Answer from the drawing. Dimensions are ordinates in mm from the lowest x, y and z of the part. A direction names the side the tool comes from. Round coordinates to 2 decimals unless told otherwise and drop trailing zeros. Write each loop counter-clockwise with the first axis right and the second up, starting at its lowest first coordinate (ties: lowest second). Pieces come first, ordered by that corner, then holes. Notation, with made-up numbers: (38.25, 17) - (78.25, 17) arc R21 ccw to (78.25, 31) - close; hole circle Ø11 at (-11.75, 54.25). An arc over 180 degrees is marked (long way). Use a Markdown table: item, result. Add a question column.
1) A tool of negligible diameter and unlimited length cuts with its end or side. For the marked faces 4, 5 and 6, from which of +Z, -Z, +X, -X, +Y, -Y can it reach the whole face along a straight path? Write none if from no direction.
2) A cutting plane is placed at A-A (x = 8.5). Give the vertices of the cut face in (y, z), then the cut area to 3 significant figures.
3) Each of these flat-tipped pins is pushed along its axis until it touches: P1, Ø2.5, axis at y = 10, z = 29, coming from the -X side; P2, Ø3, axis at x = 5, y = 4.5, coming from the +Z side; P3, Ø1, axis at y = 11, z = 26.5, coming from the +X side; P4, Ø4, axis at x = 8, z = 4, coming from the +Y side. Where does it stop, or does it pass through?
4) A cutting plane is placed at C-C (x = 4.5). Give the vertices of the cut face in (y, z), then the cut area to 3 significant figures.
5) Find the intervals of material crossed by probe 1 along Z at (x, y) = (1, 11); probe 2 along Y at (x, z) = (2.5, 20) (1 decimal); probe 3 along Z at (x, y) = (0.5, 8) (1 decimal), in increasing order. Write a range as from..to.
6) Determine the mould class of the marked faces 1, 2 and 3 for opening direction Y: +Y half, -Y half, draft (parallel to the pull), parting line (faces both ways), or undercut.
7) A cutting plane is placed at B-B (y = 9.5). State how many separate pieces and enclosed holes the cut face has.
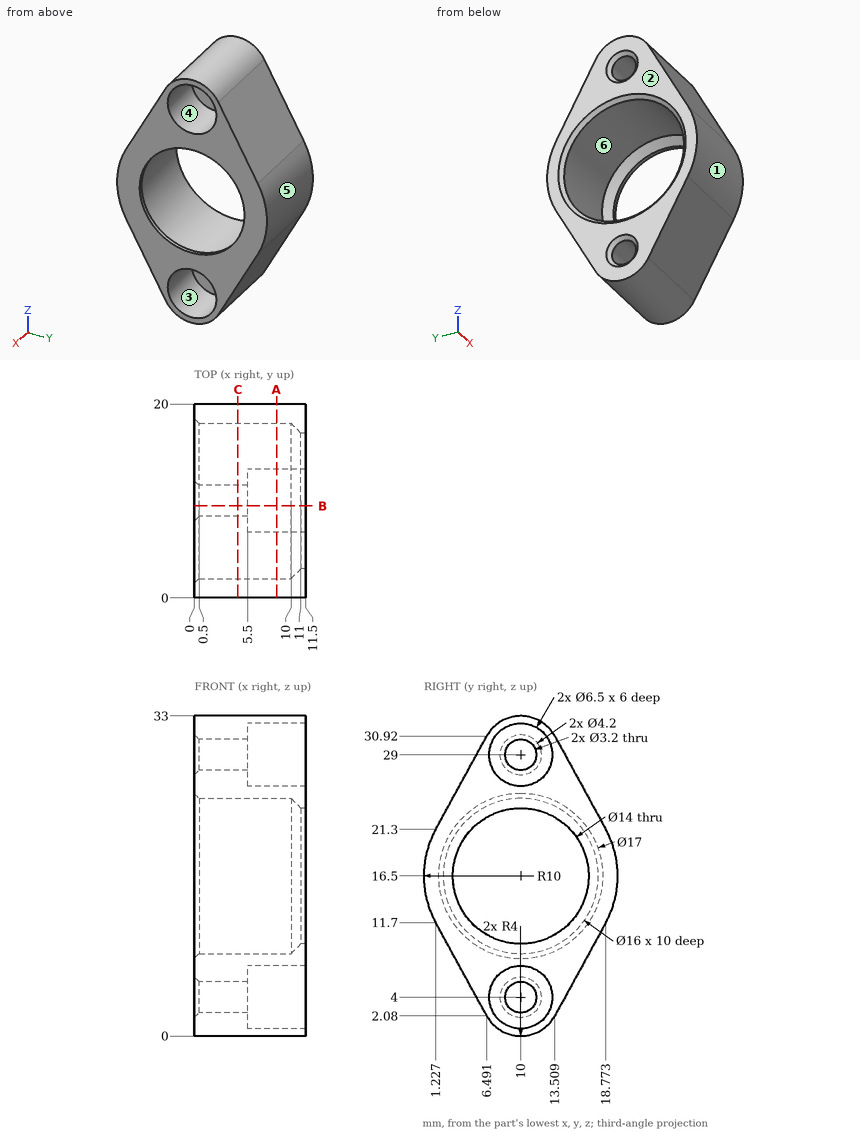
Entries:
| question | item | result |
|---|---|---|
| 1 | face 4 | +X |
| 1 | face 5 | +X, -X, +Y |
| 1 | face 6 | -X |
| 2 | outline | (1.23, 11.7) - (6.49, 2.08) arc R4 ccw to (13.51, 2.08) - (18.77, 11.7) arc R10 ccw to (18.77, 21.3) - (13.51, 30.92) arc R4 ccw to (6.49, 30.92) - (1.23, 21.3) arc R10 ccw to start; hole circle Ø16 at (10, 16.5); hole circle Ø6.5 at (10, 4); hole circle Ø6.5 at (10, 29) |
| 2 | area | 174 mm² |
| 3 | P1 | passes through |
| 3 | P2 | stops at z = 30.02 |
| 3 | P3 | stops at x = 5.5 |
| 3 | P4 | stops at y = 15.65 |
| 4 | outline | (1.23, 11.7) - (6.49, 2.08) arc R4 ccw to (13.51, 2.08) - (18.77, 11.7) arc R10 ccw to (18.77, 21.3) - (13.51, 30.92) arc R4 ccw to (6.49, 30.92) - (1.23, 21.3) arc R10 ccw to start; hole circle Ø16 at (10, 16.5); hole circle Ø3.2 at (10, 4); hole circle Ø3.2 at (10, 29) |
| 4 | area | 224 mm² |
| 5 | probe 1 | z = 0.13..2.75, 5.25..8.56, 24.44..27.75, 30.25..32.87 |
| 5 | probe 2 | y = 0.6..2.8, 17.2..19.4 |
| 5 | probe 3 | z = 0.5..8.8, 24.2..32.5 |
| 6 | face 1 | -Y half |
| 6 | face 2 | draft |
| 6 | face 3 | undercut |
| 7 | separate pieces | 4 |
| 7 | enclosed holes | 0 |
